Model file for the job. Use its own axes, mm. Face numbers are marked on the shaded views. A direction names the side the tool comes from. Coordinates: 2 decimals unless noted, no trailing zeros. Order: outer loops, then holes, each group sorted by start corner. A loop starts at its lowest first (then second) coordinate and runs counter-clockwise, first axis right, second up.
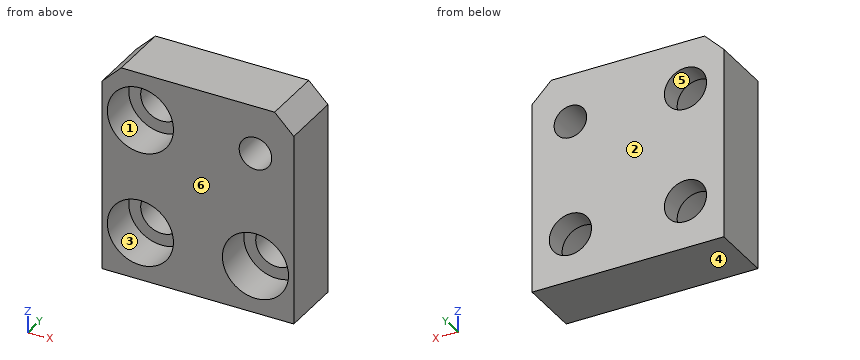
from build123d import *

# Parameters (mm, degrees)
F0_W           = 50
F0_H           = 55
F1_DEPTH       = 16
F3_D           = 11
F3_CBORE_D     = 17.25
F3_CBORE_DEPTH = 10
F5_D           = 8.5
F6_SIZE        = 5


with BuildPart() as f1:
    # F0 (on Front) → F1 (new body)
    with BuildSketch(Plane.XZ):
        Rectangle(F0_W, F0_H)
    extrude(amount=-F1_DEPTH)

    # F3 (through all)
    with Locations(Plane.XZ):
        with Locations((-15, 15), (-15, -15), (15, -15)):
            CounterBoreHole(F3_D / 2, F3_CBORE_D / 2, F3_CBORE_DEPTH)

    # F5 (through all)
    with Locations(Plane.XZ):
        with Locations((15, 15)):
            Hole(F5_D / 2)

    # F6
    f6_edges = [f1.edges().sort_by_distance(p)[0] for p in [
        (-25, 8, 27.5),
        (25, 8, 27.5),
    ]]
    chamfer(f6_edges, length=F6_SIZE)


solid = f1.part
Q1. Which spindle directions (+Z, -Z, +X, -X, +Y, -Y) get a long thin tool onto all of the face, cutting with end or side? Do the marked faces 1 and 2. Say none if no direction does.
Established:
face 1: -Y
face 2: +Z, -Z, +X, -X, +Y
Q2. Probe line 1 (Z direction, x = -15, y = 7.75) (3 decimals); line 2 (Z direction, x = -15, y = 14.05); line 3 (X direction, y = 5.25, z = -14.5). List the from-to ranges inside material, lowest first.
Established:
line 1: z = -27.5 to -23.625, -6.375 to 6.375, 23.625 to 27.5
line 2: z = -27.5 to -20.5, -9.5 to 9.5, 20.5 to 27.5
line 3: x = -25 to -23.61, -6.39 to 6.39, 23.61 to 25
Q3. Drop a flat-ended pin along its axis: P1, Ø14.5, axis at x = -15, z = -15, coming from the -Y side. Give the stop position or say it passes through.
Established:
P1: stops at y = 10
Q4. Cut at B-B, the plane z = 15. List the corners of the cut face in (x, y) (3 decimals), plus the area to 4 significant figures.
Established:
outline: (-25, 0) - (-23.625, 0) - (-23.625, 10) - (-20.5, 10) - (-20.5, 16) - (-25, 16) - close; (-9.5, 10) - (-6.375, 10) - (-6.375, 0) - (10.75, 0) - (10.75, 16) - (-9.5, 16) - close; (19.25, 0) - (25, 0) - (25, 16) - (19.25, 16) - close
area: 425.5 mm2
Q5. Cut at D-D, the plane x = 15. List the corners of the cut face in (y, z) (3 decimals).
Established:
outline: (0, -27.5) - (16, -27.5) - (16, -20.5) - (10, -20.5) - (10, -23.625) - (0, -23.625) - close; (0, -6.375) - (10, -6.375) - (10, -9.5) - (16, -9.5) - (16, 10.75) - (0, 10.75) - close; (0, 19.25) - (16, 19.25) - (16, 27.5) - (0, 27.5) - close
Q6. Cut at A-A, the plane x = -15. List the corners of the cut face in (y, z) (3 decimals).
Established:
outline: (0, -27.5) - (16, -27.5) - (16, -20.5) - (10, -20.5) - (10, -23.625) - (0, -23.625) - close; (0, -6.375) - (10, -6.375) - (10, -9.5) - (16, -9.5) - (16, 9.5) - (10, 9.5) - (10, 6.375) - (0, 6.375) - close; (0, 23.625) - (10, 23.625) - (10, 20.5) - (16, 20.5) - (16, 27.5) - (0, 27.5) - close
Q7. Mould opens along Z. For the marked faces 3, 4, 5 and 6 say: pulls with the +Z half, pulls with the -Z half, needs draft (parallel to the pull), parting line crosses it, or undercut.
Established:
face 3: undercut
face 4: pulls with the -Z half
face 5: undercut
face 6: needs draft
Q8. Cut at C-C, the plane y = 2.25. List the corners of the cut face in (x, z) (3 decimals), plus the area to 3 significant figures.
Established:
outline: (-25, -27.5) - (25, -27.5) - (25, 22.5) - (20, 27.5) - (-20, 27.5) - (-25, 22.5) - close; hole circle Ø17.25 at (-15, -15); hole circle Ø17.25 at (-15, 15); hole circle Ø17.25 at (15, -15); hole circle Ø8.5 at (15, 15)
area: 1,970 mm2
